Part model, mm, in its own coordinate system. Coordinates: 2 decimals unless noted, no trailing zeros. Loops run counter-clockwise (first coordinate to the right, second up) from the corner with the lowest first, then second, coordinate; pieces in that order, holes last. Notation, with made-up numbers: (76, 10.5) - (83, 10.5) arc R13 ccw to (83, 32.5) - close; hole circle Ø6 at (36.25, 87.5). An arc over 180 degrees is marked (long way). Use a Markdown table: item, result. Add a question column.
1. Band-saw the part on A-A, the plane y = -92.5. Give the cut face in (x, z), plus the area to 3 significant figures.
2. Band-saw the part on B-B, the plane z = 5.75. Count the separate pieces of the cut face and the enclosed holes in it, plus the area to 3 significant figures.
3. Wall check: probe 1 along Y at (x, z) = (129, 2.25); probe 2 along Y at (x, z) = (66, 2); probe 3 along Y at (x, z) = (119, 5). Give the ranges that are in metal, low to high. Write a range as [from, to].
4. Drop flat-ended pins along their axis: pin 1 (4 mm diameter, centred on x = 171.77, y = 31.77, fed in from +Z); pin 2 (2 mm diameter, centred on y = -89, z = 2, fed in from +X); pin 3 (4 mm diameter, centred on y = 26.5, z = 7, fed in from +X); pin 4 (1 mm diameter, centred on y = -48.5, z = 4.5, fed in from +X). Give the stop position or say it passes through.
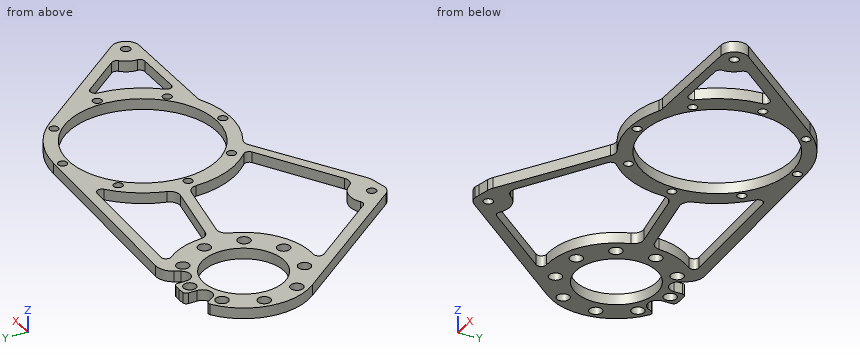
from build123d import *

# Parameters (mm, degrees)
SKETCH1_R               = 28.575
SKETCH1_R_2             = 3.29946
SKETCH1_R_3             = 9.525
SKETCH1_R_4             = 52.4256
BOSS_EXTRUDE1_DEPTH     = 7.62
CUT_EXTRUDE1_DEPTH      = 314.319493614
CUT_EXTRUDE1_DEPTH_BACK = 314.319493614
SKETCH2_R               = 4.49961
SKETCH2_R_2             = 3.175
CUT_EXTRUDE2_DEPTH      = 314.319493614
CUT_EXTRUDE2_DEPTH_BACK = 314.319493614
FILLET2_R               = 12.7
CUT_EXTRUDE3_DEPTH      = 314.319493614
CUT_EXTRUDE3_DEPTH_BACK = 314.319493614
FILLET3_R               = 2.54
FILLET4_R               = 12.7


with BuildPart() as part:
    # Sketch1 → Boss-Extrude1 (new body)
    # profile 1 of 5: a face of its own
    with BuildSketch(Plane.XY):
        with BuildLine():
            ThreePointArc((57.285987503, -118.460322704), (55.688968414, -123.739787041), (51.433442898, -127.248877555))
            Line((51.433442898, -127.248877555), (276.360987503, -82.143687357))
            ThreePointArc((276.360987503, -82.143687357), (267.780420135, -68.483534561), (283.811267218, -66.684131167))
            Line((283.811267218, -66.684131167), (220.199398147, 13.174615234))
            ThreePointArc((220.199398147, 13.174615234), (230.216497711, -4.968011872), (233.68508, -25.4))
            ThreePointArc((233.68508, -25.4), (126.817436716, -67.969857276), (175.144631834, 36.420602736))
            Line((175.144631834, 36.420602736), (5.000495975, 45.701244141))
            ThreePointArc((5.000495975, 45.701244141), (34.230844848, 30.689704088), (45.974, 0))
            ThreePointArc((45.974, 0), (15.172060928, -43.398355305), (-35.960016757, -28.644124543))
            Line((-35.960016757, -28.644124543), (40.310707788, -124.394878894))
            ThreePointArc((40.310707788, -124.394878894), (44.617604714, -109.468950749), (57.285987503, -118.460322704))
        make_face()
    # profile 2 of 5: a face of its own
    with BuildSketch(Plane.XY):
        with BuildLine():
            ThreePointArc((0, 45.974), (-41.415538495, 19.959004162), (-35.960016757, -28.644124543))
            ThreePointArc((-35.960016757, -28.644124543), (15.172060928, -43.398355305), (45.974, 0))
            ThreePointArc((45.974, 0), (34.230844848, 30.689704088), (5.000495975, 45.701244141))
            Line((5.000495975, 45.701244141), (0, 45.974))
        make_face()
        with Locations(Location((0, 0, 0), (0, 0, 180))):
            Circle(SKETCH1_R, mode=Mode.SUBTRACT)
    # profile 3 of 5: a face of its own
    with BuildSketch(Plane.XY):
        with BuildLine():
            ThreePointArc((40.310707788, -124.394878894), (43.625834707, -127.040890072), (47.760987503, -127.985322704))
            Line((47.760987503, -127.985322704), (51.433442898, -127.248877555))
            ThreePointArc((51.433442898, -127.248877555), (55.688968414, -123.739787041), (57.285987503, -118.460322704))
            ThreePointArc((57.285987503, -118.460322704), (44.617604714, -109.468950749), (40.310707788, -124.394878894))
        make_face()
        with Locations(Location((47.760987503, -118.460322704, 0), (0, 0, 180))):
            Circle(SKETCH1_R_2, mode=Mode.SUBTRACT)
    # profile 4 of 5: a face of its own
    with BuildSketch(Plane.XY):
        with Locations((276.360987503, -72.618687357)):
            Circle(SKETCH1_R_3)
        with Locations(Location((276.360987503, -72.618687357, 0), (0, 0, 180))):
            Circle(SKETCH1_R_2, mode=Mode.SUBTRACT)
    # profile 5 of 5: a face of its own
    with BuildSketch(Plane.XY):
        with BuildLine():
            ThreePointArc((233.68508, -25.4), (230.216497711, -4.968011872), (220.199398147, 13.174615234))
            ThreePointArc((220.199398147, 13.174615234), (200.160512587, 29.620750083), (175.144631834, 36.420602736))
            ThreePointArc((175.144631834, 36.420602736), (126.817436716, -67.969857276), (233.68508, -25.4))
        make_face()
        with Locations(Location((171.77258, -25.4, 0), (0, 0, 180))):
            Circle(SKETCH1_R_4, mode=Mode.SUBTRACT)
    extrude(amount=BOSS_EXTRUDE1_DEPTH)

    # Sketch2 → Cut-Extrude1 (cut, two sides: drawn at the far end of the back side and taken through both)
    with BuildSketch(Plane.XY.offset(7.62).offset(-CUT_EXTRUDE1_DEPTH_BACK)):
        with Locations((0, 38.354)):
            Circle(SKETCH2_R)
        with Locations((171.77258, 31.76905)):
            Circle(SKETCH2_R_2)
        with Locations((24.653475982, 29.380868571)):
            Circle(SKETCH2_R)
        with Locations((37.771316559, 6.660102206)):
            Circle(SKETCH2_R)
        with Locations((33.215538337, -19.177)):
            Circle(SKETCH2_R)
        with Locations((13.117840577, -36.040970778)):
            Circle(SKETCH2_R)
        with Locations((-13.117840577, -36.040970778)):
            Circle(SKETCH2_R)
        with Locations((-33.215538337, -19.177)):
            Circle(SKETCH2_R)
        with Locations((-37.771316559, 6.660102206)):
            Circle(SKETCH2_R)
        with Locations((-24.653475982, 29.380868571)):
            Circle(SKETCH2_R)
        with Locations((212.197202929, 15.024622929)):
            Circle(SKETCH2_R_2)
        with Locations((228.94163, -25.4)):
            Circle(SKETCH2_R_2)
        with Locations((212.197202929, -65.824622929)):
            Circle(SKETCH2_R_2)
        with Locations((171.77258, -82.56905)):
            Circle(SKETCH2_R_2)
        with Locations((131.347957071, -65.824622929)):
            Circle(SKETCH2_R_2)
        with Locations((114.60353, -25.4)):
            Circle(SKETCH2_R_2)
        with Locations((131.347957071, 15.024622929)):
            Circle(SKETCH2_R_2)
    extrude(amount=CUT_EXTRUDE1_DEPTH + CUT_EXTRUDE1_DEPTH_BACK, mode=Mode.SUBTRACT)

    # Sketch5 → Cut-Extrude2 (cut, two sides: drawn at the far end of the back side and taken through both)
    with BuildSketch(Plane(origin=(0, 0, 0), x_dir=(-1, 0, 0), z_dir=(0, 0, -1)).offset(-CUT_EXTRUDE2_DEPTH_BACK)):
        with BuildLine():
            ThreePointArc((-39.302161905, -105.783340827), (-36.833952554, -106.326913666), (-34.648894538, -105.056854494))
            Line((-34.648894538, -105.056854494), (6.186568412, -53.791753696))
            ThreePointArc((6.186568412, -53.791753696), (6.547130169, -50.008783233), (3.231709617, -48.151673418))
            ThreePointArc((3.231709617, -48.151673418), (-26.797926427, -40.13600303), (-45.712365207, -15.472791189))
            ThreePointArc((-45.712365207, -15.472791189), (-48.822624125, -11.670903611), (-53.666695197, -10.856633909))
            Line((-53.666695197, -10.856633909), (-101.374019125, -20.168029335))
            ThreePointArc((-101.374019125, -20.168029335), (-105.376863014, -22.522014289), (-107.019164045, -26.865613222))
            ThreePointArc((-107.019164045, -26.865613222), (-112.485034835, -51.479491719), (-126.935132299, -72.141375501))
            ThreePointArc((-126.935132299, -72.141375501), (-127.983236253, -75.050116103), (-126.302243919, -77.645026229))
            Line((-126.302243919, -77.645026229), (-69.528196733, -111.340573769))
            ThreePointArc((-69.528196733, -111.340573769), (-64.463868617, -112.307803939), (-60.115626386, -109.537290816))
            ThreePointArc((-60.115626386, -109.537290816), (-50.466052275, -103.462315351), (-39.302161905, -105.783340827))
        make_face()
        with BuildLine():
            Line((-276.360987503, -82.143687357), (-61.405360183, -125.24918816))
            Line((-61.405360183, -125.24918816), (-134.620271919, -80.665110684))
            ThreePointArc((-134.620271919, -80.665110684), (-138.295422572, -79.292203946), (-142.130961394, -80.116974938))
            ThreePointArc((-142.130961394, -80.116974938), (-169.881448075, -87.601258187), (-198.035354318, -81.816660528))
            ThreePointArc((-198.035354318, -81.816660528), (-199.517976868, -81.319553012), (-201.07403482, -81.164733259))
            Line((-201.07403482, -81.164733259), (-276.360987503, -82.143687357))
        make_face()
        with BuildLine():
            Line((-129.2329494, 31.293563157), (-40.310932114, 36.143882278))
            ThreePointArc((-40.310932114, 36.143882278), (-37.020434548, 34.248166986), (-37.423009556, 30.472052043))
            ThreePointArc((-37.423009556, 30.472052043), (-44.896236095, 17.701852573), (-48.149245066, 3.267690247))
            ThreePointArc((-48.149245066, 3.267690247), (-49.880239941, -0.880376651), (-53.780148142, -3.1149948))
            Line((-53.780148142, -3.1149948), (-101.474520552, -12.423862382))
            ThreePointArc((-101.474520552, -12.423862382), (-106.457644943, -11.526726906), (-109.525506814, -7.498749212))
            ThreePointArc((-109.525506814, -7.498749212), (-117.850437324, 10.482522615), (-131.222021432, 25.105495738))
            ThreePointArc((-131.222021432, 25.105495738), (-132.356283928, 28.883803437), (-129.2329494, 31.293563157))
        make_face()
        with BuildLine():
            ThreePointArc((-243.589980451, -28.420218982), (-239.843636661, -27.262743932), (-237.398113791, -30.327749345))
            ThreePointArc((-237.398113791, -30.327749345), (-232.320070073, -51.187493962), (-220.7984065, -69.302867047))
            ThreePointArc((-220.7984065, -69.302867047), (-220.204512197, -73.023273129), (-223.345463701, -75.103791216))
            Line((-223.345463701, -75.103791216), (-257.603993865, -75.549253906))
            ThreePointArc((-257.603993865, -75.549253906), (-260.057201806, -74.581862154), (-261.127541325, -72.171789682))
            ThreePointArc((-261.127541325, -72.171789682), (-262.4556706, -66.381719999), (-265.89655065, -61.539284785))
            ThreePointArc((-265.89655065, -61.539284785), (-266.978290112, -59.255128799), (-266.229006424, -56.84139667))
            Line((-266.229006424, -56.84139667), (-243.589980451, -28.420218982))
        make_face()
    extrude(amount=CUT_EXTRUDE2_DEPTH + CUT_EXTRUDE2_DEPTH_BACK, mode=Mode.SUBTRACT)

    # Fillet2
    fillet2_edges = [part.edges().sort_by_distance(p)[0] for p in [
        (61.405360183, -125.24918816, 3.81),
    ]]
    fillet(fillet2_edges, radius=FILLET2_R)

    # Sketch6 → Cut-Extrude3 (cut, two sides: drawn at the far end of the back side and taken through both)
    with BuildSketch(Plane(origin=(0, 0, 0), x_dir=(-1, 0, 0), z_dir=(0, 0, -1)).offset(-CUT_EXTRUDE3_DEPTH_BACK)):
        with BuildLine():
            Line((-19.149599026, 33.871202127), (-25.180470346, 44.600512078))
            Line((-25.180470346, 44.600512078), (-6.983635222, 45.593072301))
            Line((-6.983635222, 45.593072301), (-6.983635222, 37.0560801))
            ThreePointArc((-6.983635222, 37.0560801), (-11.837393988, 30.76811296), (-19.149599026, 33.871202127))
        make_face()
        with BuildLine():
            Line((6.694264778, 36.870190043), (6.694264778, 45.484013621))
            ThreePointArc((6.694264778, 45.484013621), (15.174774423, 43.397406572), (23.107677895, 39.744734221))
            Line((23.107677895, 39.744734221), (19.260113276, 33.371320679))
            ThreePointArc((19.260113276, 33.371320679), (11.648320448, 30.348253304), (6.694264778, 36.870190043))
        make_face()
    extrude(amount=CUT_EXTRUDE3_DEPTH + CUT_EXTRUDE3_DEPTH_BACK, mode=Mode.SUBTRACT)

    # Fillet3
    fillet3_edges = [part.edges().sort_by_distance(p)[0] for p in [
        (-6.694264778, 45.484013621, 3.81),
        (6.983635222, 45.593072301, 3.81),
        (-23.107677895, 39.744734221, 3.81),
    ]]
    fillet(fillet3_edges, radius=FILLET3_R)

    # Fillet4
    fillet4_edges = [part.edges().sort_by_distance(p)[0] for p in [
        (25.180470346, 44.600512078, 3.81),
    ]]
    fillet(fillet4_edges, radius=FILLET4_R)


solid = part.part
Geometry check:
| question | item | result |
|---|---|---|
| 1 | outline | (14.9, 0) - (24.65, 0) - (24.65, 7.62) - (14.9, 7.62) - close; (101.27, 0) - (115.19, 0) - (115.19, 7.62) - (101.27, 7.62) - close |
| 1 | area | 180 mm^2 |
| 2 | separate pieces | 1 |
| 2 | enclosed holes | 24 |
| 2 | area | 12,000 mm^2 |
| 3 | probe 1 | y = [-84.09, -67.96], [-63.69, -55.71], [4.91, 12.89], [17.16, 23.24], [31.31, 38.94] |
| 3 | probe 2 | y = [-122.45, -112.43], [-13.26, -5.5], [34.74, 42.37] |
| 3 | probe 3 | y = [-90.18, -81.98], [-62.95, 12.15], [31.85, 39.48] |
| 4 | pin 1 | passes through |
| 4 | pin 2 | stops at x = 122.58 |
| 4 | pin 3 | stops at x = 208.42 |
| 4 | pin 4 | stops at x = 269.72 |
